Geometry check sheet. Reference: the model listing, model coordinates, mm. Give positions to 0.01 mm unless a question says otherwise; leave off trailing zeros. Write each loop counter-clockwise with the first axis right and the second up, starting at its lowest first coordinate (ties: lowest second). Pieces come first, ordered by that corner, then holes. Notation, with made-up numbers: (-39.75, 39.5) -> (13.25, 39.5) arc R14 ccw to (13.25, 53.5) -> close; hole circle Ø2 at (31.25, -13). An arc over 180 degrees is marked (long way). Write item = value, one per line. Start each with the question number.
1. Cross-section at B-B, the plane z = 15.24. Record the cut outline in (x, y).
2. Cross-section at C-C, the plane x = 0. Record the cut outline in (y, z).
3. Thickness scan on line 1 along X through (y, z) = (0.5, 15.24); line 2 along X through (y, z) = (0.6, 16.5); line 3 along Z through (x, y) = (-1, 0.4). Record the ranges inside material, lowest first.
4. Cross-section at D-D, the plane y = 0.3. Record the cut outline in (x, z) (3 decimals).
5. Cross-section at A-A, the plane x = -10.16. Record the cut outline in (y, z).
6. Depth check by flat-ended pin: P1, Ø3, axis at x = -10.16, z = -15.24, coming from the +Y side. Enter the tip coordinate at first touch or a pass-through.
```python
from build123d import *

# Parameters (mm, degrees)
SKETCH1_W           = 30.48
SKETCH1_H           = 38.1
SKETCH1_R           = 1.778
BOSS_EXTRUDE1_DEPTH = 1.27
SKETCH2_R           = 1.778
SKETCH2_R_2         = 1.905
CUT_EXTRUDE1_DEPTH  = 25.428937758


with BuildPart() as part:
    # Sketch1 → Boss-Extrude1 (new body)
    with BuildSketch(Plane(origin=(0, 0, 0), x_dir=(1, 0, 0), z_dir=(0, 1, 0))):
        Rectangle(SKETCH1_W, SKETCH1_H)
        with Locations(Location((-10.16, 15.24, 0), (0, 0, 270))):
            Circle(SKETCH1_R, mode=Mode.SUBTRACT)
        with Locations(Location((10.16, 15.24, 0), (0, 0, 90))):
            Circle(SKETCH1_R, mode=Mode.SUBTRACT)
        with Locations(Location((-10.16, -15.24, 0), (0, 0, 90))):
            Circle(SKETCH1_R, mode=Mode.SUBTRACT)
        with Locations(Location((10.16, -15.24, 0), (0, 0, 270))):
            Circle(SKETCH1_R, mode=Mode.SUBTRACT)
    extrude(amount=BOSS_EXTRUDE1_DEPTH)

    # Sketch2 → Cut-Extrude1 (cut, through all)
    with BuildSketch(Plane.XZ):
        with Locations(Location((-10.16, -15.24, 0), (0, 0, 90))):
            Circle(SKETCH2_R)
        with Locations(Location((10.16, -15.24, 0), (0, 0, 270))):
            Circle(SKETCH2_R)
        with Locations(Location((10.16, 15.24, 0), (0, 0, 90))):
            Circle(SKETCH2_R)
        with Locations(Location((-10.16, 15.24, 0), (0, 0, 270))):
            Circle(SKETCH2_R)
        with Locations(Location((0, -1.5494, 0), (0, 0, 270))):
            Circle(SKETCH2_R_2)
    extrude(amount=-CUT_EXTRUDE1_DEPTH, mode=Mode.SUBTRACT)


solid = part.part
```
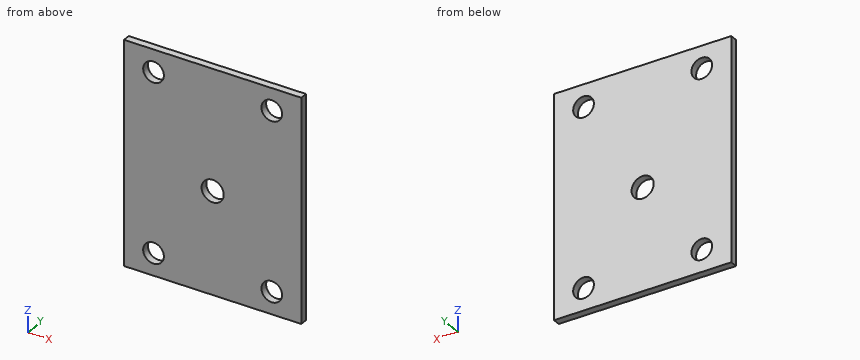
Answers:
q1.outline = (-15.24, 0) -> (-11.94, 0) -> (-11.94, 1.27) -> (-15.24, 1.27) -> close; (-8.38, 0) -> (8.38, 0) -> (8.38, 1.27) -> (-8.38, 1.27) -> close; (11.94, 0) -> (15.24, 0) -> (15.24, 1.27) -> (11.94, 1.27) -> close
q2.outline = (0, -19.05) -> (1.27, -19.05) -> (1.27, -3.45) -> (0, -3.45) -> close; (0, 0.36) -> (1.27, 0.36) -> (1.27, 19.05) -> (0, 19.05) -> close
q3.line_1 = -15.24 to -11.94, -8.38 to 8.38, 11.94 to 15.24
q3.line_2 = -15.24 to -11.41, -8.91 to 8.91, 11.41 to 15.24
q3.line_3 = -19.05 to -3.17, 0.07 to 19.05
q4.outline = (-15.24, -19.05) -> (15.24, -19.05) -> (15.24, 19.05) -> (-15.24, 19.05) -> close; hole circle Ø3.556 at (-10.16, -15.24); hole circle Ø3.556 at (-10.16, 15.24); hole circle Ø3.81 at (0, -1.549); hole circle Ø3.556 at (10.16, -15.24); hole circle Ø3.556 at (10.16, 15.24)
q5.outline = (0, -19.05) -> (1.27, -19.05) -> (1.27, -17.02) -> (0, -17.02) -> close; (0, -13.46) -> (1.27, -13.46) -> (1.27, 13.46) -> (0, 13.46) -> close; (0, 17.02) -> (1.27, 17.02) -> (1.27, 19.05) -> (0, 19.05) -> close
q6.P1 = through
